Autodesk Inventor part; units mm, degrees
ref_plane "YZ Plane" through (0, 0, 0) normal (1, 0, 0) x (0, 1, 0)
ref_plane "XZ Plane" through (0, 0, 0) normal (0, 1, 0) x (-1, 0, 0)
ref_plane "XY Plane" through (0, 0, 0) normal (0, 0, 1) x (1, 0, 0)
sketch "Boceto1" plane through (0, 0, 0) normal (0, 0, 1) x (1, 0, 0)
  line L0 (-24.1261, 0) -> (26.0802, 0) construction
  line L1 (0, 10.125) -> (-30, 10.125)
  line L2 (-30, 10.125) -> (-30, 15)
  line L3 (-30, 15) -> (-15, 15)
  line L4 (-15, 15) -> (-15, 31)
  line L5 (0, 31) -> (0, 10.125)
  line L6 (-15, 31) -> (-13, 31)
  line L7 (-13, 31) -> (-10, 27.5)
  line L8 (-10, 27.5) -> (-5, 27.5)
  line L9 (-2, 31) -> (0, 31)
  line L10 (-2, 31) -> (-5, 27.5)
  line L11 (-7.5, 27.5) -> (-7.5, 0) construction
  point P0 (0, 0)
  point P1 (0, 20.5625)
  dimension "d0" = 27.5
  dimension "d1" = 31
  dimension "d2" = 10.125
  dimension "d3" = 15
  dimension "d4" = 15
  dimension "d5" = 2
  dimension "d6" = 2
  dimension "d7" = 5
  dimension "d8" = 7.5
  dimension "d9" = 15
revolve "Revolución1" add sketch "Boceto1" angle 360 about axis through (-24.1261, 0, 0) along (1, 0, 0)
properties part number "PoleaBrazos"
Verification items for the finished model (mm, model axes). A direction names the side the tool comes from. Round coordinates to 2 decimals unless told otherwise and drop trailing zeros. Order: outer loops, then holes, each group sorted by start corner. A loop starts at its lowest first (then second) coordinate and runs counter-clockwise, first axis right, second up. Notation, with made-up numbers: (-33, 37.5) - (16, 37.5) arc R21 cw to (16, 53.5) - close; hole circle Ø5 at (52, 53.25). An arc over 180 degrees is marked (long way). Use CSV: the item, a comma, the result in double quotes.
(1) Section check C-C on x = -8.25. Record the boundary of the cut face in (y, z) (3 decimals).
Entries:
outline,"circle Ø55 at (0, 0); hole circle Ø20.25 at (0, 0)"
(2) Mould release check, pull along Z, two halves, no side actions. Record for faces 1 (the face through (-0.986, -4.036, 30.736)), 2 (the face through (-30, 3, -10)), 3 (the face through (-15.21, 5.44, -8.54)): released by +Z, released by -Z, zero draft, split by the parting line, or undercut.
Entries:
face 1,"split by the parting line"
face 2,"zero draft"
face 3,"undercut"
(3) Access from +Z, -Z, +X, -X, +Y, -Y to the whole of each face (thin tool, end or side, straight path). Record for faces 4 (the face through (-15, 13.3, 7.3)), 5 (the face through (-13.986, -4.036, 30.736)), 6 (the face through (-4.81, -22, -16.87)).
Entries:
face 4,"-X"
face 5,"+X, -X"
face 6,"none"
(4) Gauge pin test, flat ends, axial feed: pin 1 Ø1.5 at (y, z) = (21.5, -11) entering from -X; pin 2 Ø4 at (x, z) = (-7.5, -9) entering from -Y; pin 3 Ø4 at (x, z) = (-21.5, -3) entering from -Y. Record the tip position at first contact, or that the pin passes through.
Entries:
pin 1,"x = -15"
pin 2,"y = -26.59"
pin 3,"y = -14.97"
(5) Thickness scan on probe 1 along Z at (x, y) = (-23.25, 0) (3 decimals); probe 2 along Z at (x, y) = (-13, 0) (3 decimals); probe 3 along X at (y, z) = (19, 2). Record the ranges inside material, lowest first. Write a range as from..to.
Entries:
probe 1,"-15..-10.125, 10.125..15"
probe 2,"-31..-10.125, 10.125..31"
probe 3,"-15..0"
(6) Section check A-A on y = 0. Record the boundary of the cut face in (x, z) (3 decimals), and give its area (4 significant figures).
Entries:
outline,"(-30, -15) - (-15, -15) - (-15, -31) - (-13, -31) - (-10, -27.5) - (-5, -27.5) - (-2, -31) - (0, -31) - (0, -10.125) - (-30, -10.125) - close; (-30, 10.125) - (0, 10.125) - (0, 31) - (-2, 31) - (-5, 27.5) - (-10, 27.5) - (-13, 31) - (-15, 31) - (-15, 15) - (-30, 15) - close"
area,"716.5 mm^2"
